The figure shows three views and two pictorial views of one solid part (mm, origin at its lowest corner). Answer the questions. Round coordinates to 2 decimals unless told otherwise and drop trailing zeros. Write each loop counter-clockwise with the first axis right and the second up, starting at its lowest first coordinate (ties: lowest second). Pieces come first, ordered by that corner, then holes.
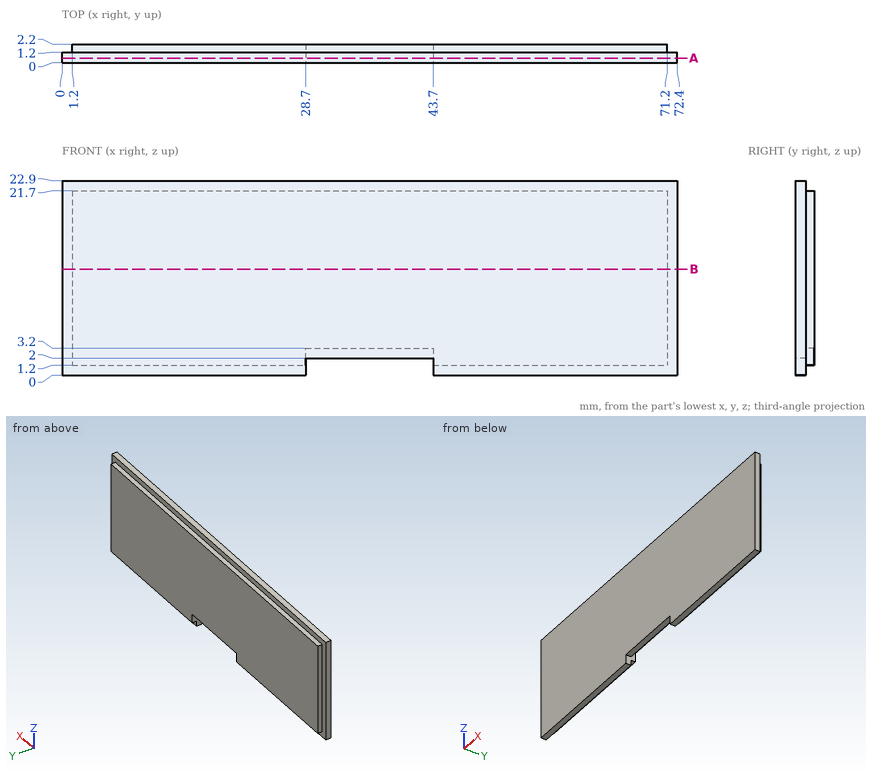
Q1. Section B-B (z = 12.5) is taken. Determine the outline of the cut face in (x, y).
Verdict:
outline: (0, 0) - (72.4, 0) - (72.4, 1.2) - (71.2, 1.2) - (71.2, 2.2) - (1.2, 2.2) - (1.2, 1.2) - (0, 1.2) - close
Q2. Flat-ended cylindrical pins translate along their axes: pin 1 Ø1.3 at (x, y) = (35.5, 0.5) entering from -Z; pin 2 Ø0.5 at (y, z) = (2, 16) entering from +X; pin 3 Ø0.5 at (x, y) = (22.5, 1.5) entering from +Z. Find the tip coordinate at first contact, or state that the pin passes through.
Verdict:
pin 1: stops at z = 2
pin 2: stops at x = 71.2
pin 3: stops at z = 21.7
Q3. Straight lines are drawn through the part: probe 1 along Z at (x, y) = (69, 1.5); probe 2 along X at (y, z) = (1.65, 2.75); probe 3 along X at (y, z) = (1.45, 12.5). For each, find the intervals that lie inside material, in ascending order.
Verdict:
probe 1: z = 1.2 to 21.7
probe 2: x = 1.2 to 28.7, 43.7 to 71.2
probe 3: x = 1.2 to 71.2
Q4. Section A-A (y = 0.55) is taken. Determine the outline of the cut face in (x, z).
Verdict:
outline: (0, 0) - (28.7, 0) - (28.7, 2) - (43.7, 2) - (43.7, 0) - (72.4, 0) - (72.4, 22.9) - (0, 22.9) - close
